Autodesk Inventor part; units mm, degrees
ref_plane "YZ Plane" through (0, 0, 0) normal (1, 0, 0) x (0, 1, 0)
ref_plane "XZ Plane" through (0, 0, 0) normal (0, 1, 0) x (-1, 0, 0)
ref_plane "XY Plane" through (0, 0, 0) normal (0, 0, 1) x (1, 0, 0)
sketch "Sketch1" plane through (0, 0, 0) normal (0, 1, 0) x (-1, 0, 0)
  line L0 (0, 0) -> (3, 0)
  line L1 (3, 0) -> (3, -25)
  line L2 (3, -25) -> (0, -25)
  line L3 (0, -25) -> (0, 0)
  line L4 (8.2, 0) -> (11.2, 0)
  line L5 (11.2, 0) -> (11.2, -25)
  line L6 (11.2, -25) -> (8.2, -25)
  line L7 (8.2, -25) -> (8.2, 0)
  point P0 (0, -12.5)
  point P1 (8.2, -12.5)
  dimension "d0" = 25
  dimension "d1" = 3
  dimension "d2" = 25
  dimension "d3" = 3
  dimension "d4" = 5.2
extrude "Extrusion1" add sketch "Sketch1" along normal blind 15
sketch "Sketch2" plane through (0, 15, 0) normal (0, 1, 0) x (1, 0, 0)
  line L0 (-11.2, 25) -> (-11.2, 0)
  line L1 (-11.2, 0) -> (0, 0)
  line L2 (0, 0) -> (0, 25)
  line L3 (0, 25) -> (-11.2, 25)
  line L4 (-11.2, 25) -> (-11.2, 0)
  point P0 (0, 0)
extrude "Extrusion2" add sketch "Sketch2" along normal blind 10
sketch "Sketch3" plane through (0, 0, 0) normal (1, 0, 0) x (0, 0, -1)
  line L0 (0, 25) -> (25, 25)
  line L1 (12.5, 25) -> (12.5, 0.2306)
  line L2 (9.5, 25) -> (9.5, 21)
  line L3 (9.5, 21) -> (7.8272, 21)
  line L4 (7.8272, 21) -> (7.8272, 16)
  line L5 (7.8272, 16) -> (12.5, 16)
  line L6 (15.5, 25) -> (15.5, 21)
  line L7 (15.5, 21) -> (17.1728, 21)
  line L8 (17.1728, 21) -> (17.1728, 16)
  line L9 (17.1728, 16) -> (12.5, 16)
  line L10 (9.5, 25) -> (15.5, 25)
  circle A0 centre (12.5, 3.7087) radius 2.6
  point P0 (0, 0)
  point P1 (8.6636, 21)
  dimension "d9" = 6
  dimension "d10" = 5
  dimension "d11" = 8
  dimension "d14" = 5.2
extrude "Extrusion3" cut sketch "Sketch3" against normal blind 20
properties part number "RollYAxisEnd" material "Thermoplastic Resin"
Here's how the part is built. I have some questions about the finished solid (model axes, mm). A direction names the side the tool comes from. Coordinates: 2 decimals unless noted, no trailing zeros. Write each loop counter-clockwise with the first axis right and the second up, starting at its lowest first coordinate (ties: lowest second). Pieces come first, ordered by that corner, then holes.
Item 1: I want a section at A-A on z = -12.5. Write out the boundary of the cut face in (x, y), and give its area (3 significant figures).
Item 2: Will these pins go through, and if not, where does the flat tip stop? pin 1 (1.8 mm diameter, centred on x = -4, z = -16.5, fed in from -Y); pin 2 (1 mm diameter, centred on x = -4, y = 14, fed in from -Z).
Item 3: If we mould it in two halves opening along X, with no side actions, what happens to faces 6 (the flat face through (-6, 15, -13)), 7 (the flat face through (0, 12, -12)), 8 (the flat face through (-8.2, 7, -13)), 9 (the flat face through (-6, 18, -25))? For each: +X half, -X half, draft (parallel to the pull), parting line (faces both ways), or undercut.
Item 4: If I drill on line 1 (Z direction, x = -6.5, y = 22.75); line 2 (X direction, y = 10.75, z = -2); line 3 (Y direction, x = -9.9, z = -12.5), over which ranges is the centre line in solid material (lowest first)?
Item 5: On a 3-axis mill with a long thin cutter (end or side, diameter ignored), from which of +Z, -Z, +X, -X, +Y, -Y can I reach the whole of each face in a straight line? I mean faces 1 (the flat face through (-6, 23, -9.5)), 2 (the flat face through (-3, 7, -12)), 3 (the flat face through (-6, 25, -20)), 4 (the flat face through (-6, 16, -12)), 5 (the flat face through (-11.2, 12, -13)). Say none if no direction works.
Item 6: I want a section at B-B on y = 21.75. Write out the boundary of the cut face in (x, z), and give its area (3 significant figures).
Item 7: I want a section at C-C on z = -8.5. Write out the boundary of the cut face in (x, y).
Item 8: I want a section at D-D on x = -6.5. Write out the boundary of the cut face in (y, z), and give its area (3 significant figures).
Findings below:
1. outline: (-11.2, 0) - (-8.2, 0) - (-8.2, 1.11) - (-11.2, 1.11) - close; (-11.2, 6.31) - (-8.2, 6.31) - (-8.2, 15) - (-3, 15) - (-3, 6.31) - (0, 6.31) - (0, 16) - (-11.2, 16) - close; (-3, 0) - (0, 0) - (0, 1.11) - (-3, 1.11) - close
1. area: 70.0 mm2
2. pin 1: stops at y = 15
2. pin 2: passes through
3. face 6: undercut
3. face 7: +X half
3. face 8: undercut
3. face 9: draft
4. line 1: z = -25 to -15.5, -9.5 to 0
4. line 2: x = -11.2 to -8.2, -3 to 0
4. line 3: y = 0 to 1.11, 6.31 to 16
5. face 1: +X, -X, +Y
5. face 2: +Z, -Z, -Y
5. face 3: +Z, -Z, +X, -X, +Y
5. face 4: +X, -X
5. face 5: +Z, -Z, -X, +Y, -Y
6. outline: (-11.2, -25) - (0, -25) - (0, -15.5) - (-11.2, -15.5) - close; (-11.2, -9.5) - (0, -9.5) - (0, 0) - (-11.2, 0) - close
6. area: 213 mm2
7. outline: (-11.2, 0) - (-8.2, 0) - (-8.2, 15) - (-3, 15) - (-3, 0) - (0, 0) - (0, 16) - (-11.2, 16) - close; (-11.2, 21) - (0, 21) - (0, 25) - (-11.2, 25) - close
8. outline: (15, -25) - (25, -25) - (25, -15.5) - (21, -15.5) - (21, -17.17) - (16, -17.17) - (16, -7.83) - (21, -7.83) - (21, -9.5) - (25, -9.5) - (25, 0) - (15, 0) - close
8. area: 179 mm2
